For this review, take the finished solid that the model builds, in its own axes (mm). A direction names the side the tool comes from. Give positions to 0.01 mm unless a question says otherwise; leave off trailing zeros. Write each loop counter-clockwise with the first axis right and the second up, starting at its lowest first coordinate (ties: lowest second). Pieces come first, ordered by that corner, then holes. Notation, with made-up numbers: M 20,-29.5 L 77,-29.5 A16 ccw 77,-25.5 Z; hole C 55.25,78.5 d6. An arc over 180 degrees is marked long. Write item = value, one per line.
```python
from build123d import *

# Parameters (mm, degrees)
SKETCH2_W           = 54.6
SKETCH2_H           = 28
SKETCH2_R           = 2.04
SKETCH2_W_2         = 40.6
SKETCH2_H_2         = 20.5
BOSS_EXTRUDE1_DEPTH = 7.5
BOSS_EXTRUDE2_DEPTH = 7.5
BOSS_EXTRUDE3_DEPTH = 40.72
SKETCH6_W           = 18.087587328
SKETCH6_H           = 12.11
SKETCH6_W_2         = 10.871882737
CUT_EXTRUDE2_DEPTH  = 75
CUT_EXTRUDE3_DEPTH  = 24.22
FILLET2_START       = -28.72
FILLET2_DEPTH       = 24.22
FILLET2_START_2     = -3.36744
FILLET2_2_DEPTH     = 11.36744
FILLET2_START_3     = -40.72
FILLET2_3_DEPTH     = 12
FILLET2_START_4     = -4.5
FILLET2_4_DEPTH     = 12
FILLET3_R           = 2
SKETCH8_W           = 25
SKETCH8_H           = 9
SKETCH8_R           = 2.05
BOSS_EXTRUDE4_DEPTH = 7.5
BOSS_EXTRUDE5_DEPTH = 18.75
FILLET5_START       = -59.47
FILLET5_DEPTH       = 18.75
FILLET5_START_2     = -40.72
FILLET5_2_DEPTH     = 12
FILLET5_START_3     = -28.72
FILLET5_3_DEPTH     = 36.72
SKETCH10_R          = 2.05
CUT_EXTRUDE4_DEPTH  = 48.75
SKETCH11_R          = 2.05
CUT_EXTRUDE5_DEPTH  = 13.75


with BuildPart() as part:
    # Sketch2 → Boss-Extrude1 (new body)
    with BuildSketch(Plane.XY):
        Rectangle(SKETCH2_W, SKETCH2_H)
        with Locations((23.85, 4.9)):
            Circle(SKETCH2_R, mode=Mode.SUBTRACT)
        with Locations((23.85, -4.9)):
            Circle(SKETCH2_R, mode=Mode.SUBTRACT)
        with Locations((-23.85, -4.9)):
            Circle(SKETCH2_R, mode=Mode.SUBTRACT)
        with Locations((-23.85, 4.9)):
            Circle(SKETCH2_R, mode=Mode.SUBTRACT)
        Rectangle(SKETCH2_W_2, SKETCH2_H_2, mode=Mode.SUBTRACT)
    extrude(amount=BOSS_EXTRUDE1_DEPTH)

    # Sketch3 → Boss-Extrude2 (add)
    with BuildSketch(Plane.XY.offset(7.5)):
        with BuildLine():
            ThreePointArc((60.895347856, 47.266361721), (62.080408935, 46.696685397), (63.247918809, 46.091853548))
            Line((63.247918809, 46.091853548), (65.410652729, 47.340508558))
            ThreePointArc((65.410652729, 47.340508558), (63.367825291, 52.693526286), (60.533352794, 57.672854393))
            ThreePointArc((60.533352794, 57.672854393), (14.45073797, 52.932517239), (-10.655780842, 14))
            Line((-10.655780842, 14), (27.3, 14))
            Line((27.3, 14), (29.456139987, 36.685790659))
            ThreePointArc((29.456139987, 36.685790659), (31.415329504, 44.731485751), (36.854221074, 50.975690388))
            ThreePointArc((36.854221074, 50.975690388), (38.81261709, 52.175562601), (40.911281353, 53.108630977))
            Line((40.911281353, 53.108630977), (43.979720969, 47.793937662))
            Line((43.979720969, 47.793937662), (43.979720969, 53.930816894))
            ThreePointArc((43.979720969, 53.930816894), (53.370921787, 52.967700083), (60.895347856, 47.266361721))
        make_face()
        with BuildLine():
            ThreePointArc((0.216101895, 19.75), (7.968248239, 34.690697157), (20.76316619, 45.627345599))
            Line((20.76316619, 45.627345599), (18.303689223, 19.75))
            Line((18.303689223, 19.75), (0.216101895, 19.75))
        make_face(mode=Mode.SUBTRACT)
    extrude(amount=-BOSS_EXTRUDE2_DEPTH)

    # Sketch4 → Boss-Extrude3 (add)
    with BuildSketch(Plane(origin=(0, 0, 0), x_dir=(-1, 0, 0), z_dir=(0, 0, -1))):
        with BuildLine():
            Line((-27.3, 14), (10.655780842, 14))
            ThreePointArc((10.655780842, 14), (-14.45073797, 52.932517239), (-60.533352794, 57.672854393))
            ThreePointArc((-60.533352794, 57.672854393), (-63.367825291, 52.693526286), (-65.410652729, 47.340508558))
            Line((-65.410652729, 47.340508558), (-63.247918809, 46.091853548))
            ThreePointArc((-63.247918809, 46.091853548), (-62.080408935, 46.696685397), (-60.895347856, 47.266361721))
            ThreePointArc((-60.895347856, 47.266361721), (-53.370921787, 52.967700083), (-43.979720969, 53.930816894))
            Line((-43.979720969, 53.930816894), (-43.979720969, 47.793937662))
            Line((-43.979720969, 47.793937662), (-40.911281353, 53.108630977))
            ThreePointArc((-40.911281353, 53.108630977), (-32.60282981, 46.697408258), (-29.456139987, 36.685790659))
            Line((-29.456139987, 36.685790659), (-27.3, 14))
        make_face()
        with BuildLine():
            ThreePointArc((-20.76316619, 45.627345599), (-7.968248239, 34.690697157), (-0.216101895, 19.75))
            Line((-0.216101895, 19.75), (-18.303689223, 19.75))
            Line((-18.303689223, 19.75), (-20.76316619, 45.627345599))
        make_face(mode=Mode.SUBTRACT)
    extrude(amount=BOSS_EXTRUDE3_DEPTH)

    # Sketch6 → Cut-Extrude2 (cut)
    with BuildSketch(Plane.XZ.offset(-14)):
        with Locations((9.259895559, -22.665)):
            Rectangle(SKETCH6_W, SKETCH6_H)
        with Locations((9.259895559, -10.555)):
            Rectangle(SKETCH6_W, SKETCH6_H)
        with Locations((-5.219839474, -10.555)):
            Rectangle(SKETCH6_W_2, SKETCH6_H)
        with Locations((-5.219839474, -22.665)):
            Rectangle(SKETCH6_W_2, SKETCH6_H)
    extrude(amount=-CUT_EXTRUDE2_DEPTH, mode=Mode.SUBTRACT)

    # Sketch7 → Cut-Extrude3 (cut)
    with BuildSketch(Plane(origin=(0, 0, -4.5), x_dir=(-1, 0, 0), z_dir=(0, 0, -1))):
        Polygon((-18.303689223, 19.75), (-27.846500896, 19.75), (-54.079071881, 47.777058416), (-54.079071881, 65.656726539), (-18.303689223, 62.002487799), align=None)
    extrude(amount=CUT_EXTRUDE3_DEPTH, mode=Mode.SUBTRACT)

    # Fillet2: read off the stored shape, not the designer's step
    # Fillet2 outline → Fillet2 (cut)
    with BuildSketch(Plane.XY.offset(FILLET2_START)):
        with BuildLine():
            ThreePointArc((55.143386559, 52.15249663), (54.365687709, 52.888463891), (54.079071881, 53.920120169))
            Line((54.079071881, 53.920120169), (54.079071881, 52.670590979))
            ThreePointArc((54.079071881, 52.670590979), (54.615611027, 52.420545294), (55.143386559, 52.15249663))
        make_face()
        with BuildLine():
            ThreePointArc((56.609256937, 58.915929333), (55.348001268, 59.246208749), (54.079071881, 59.545655852))
            Line((54.079071881, 59.545655852), (54.079071881, 56.987483377))
            ThreePointArc((54.079071881, 56.987483377), (54.866712634, 58.57813892), (56.609256937, 58.915929333))
        make_face()
        with BuildLine():
            Line((18.303689223, 19.75), (18.303689223, 17.75))
            ThreePointArc((18.303689223, 17.75), (18.88947566, 19.164213562), (20.303689223, 19.75))
            Line((20.303689223, 19.75), (18.303689223, 19.75))
        make_face()
    extrude(amount=FILLET2_DEPTH, mode=Mode.SUBTRACT)

    # Fillet2 2 outline → Fillet2 2 (cut)
    with BuildSketch(Plane.XY.offset(FILLET2_START_2)):
        with BuildLine():
            Line((-27.3, 14), (-27.3, 12))
            ThreePointArc((-27.3, 12), (-26.714213562, 13.414213562), (-25.3, 14))
            Line((-25.3, 14), (-27.3, 14))
        make_face()
        with BuildLine():
            ThreePointArc((27.3, -12), (26.714213562, -13.414213562), (25.3, -14))
            Line((25.3, -14), (27.3, -14))
            Line((27.3, -14), (27.3, -12))
        make_face()
    extrude(amount=FILLET2_2_DEPTH, mode=Mode.SUBTRACT)

    # Fillet2 3 outline → Fillet2 3 (add)
    with BuildSketch(Plane.XY.offset(FILLET2_START_3)):
        with BuildLine():
            ThreePointArc((17.242809806, 43.409998621), (19.395297177, 43.497545876), (20.378564388, 41.5807642))
            Line((20.378564388, 41.5807642), (20.76316619, 45.627345599))
            ThreePointArc((20.76316619, 45.627345599), (18.976765346, 44.560304331), (17.242809806, 43.409998621))
        make_face()
    extrude(amount=FILLET2_3_DEPTH)

    # Fillet2 4 outline → Fillet2 4 (add)
    with BuildSketch(Plane.XY.offset(FILLET2_START_4)):
        with BuildLine():
            ThreePointArc((17.242809806, 43.409998621), (19.395297177, 43.497545876), (20.378564388, 41.5807642))
            Line((20.378564388, 41.5807642), (20.76316619, 45.627345599))
            ThreePointArc((20.76316619, 45.627345599), (18.976765346, 44.560304331), (17.242809806, 43.409998621))
        make_face()
    extrude(amount=FILLET2_4_DEPTH)

    # Fillet3
    fillet3_edges = [part.edges().sort_by_distance(p)[0] for p in [
        (-10.655780842, 14, 3.75),
    ]]
    fillet(fillet3_edges, radius=FILLET3_R)

    # Sketch8 → Boss-Extrude4 (add)
    with BuildSketch(Plane(origin=(0, 0, 0), x_dir=(-1, 0, 0), z_dir=(0, 0, -1))):
        with Locations((14.8, -18.5)):
            Rectangle(SKETCH8_W, SKETCH8_H)
        with Locations((19.8, -18.5)):
            Circle(SKETCH8_R, mode=Mode.SUBTRACT)
        with Locations(Location((9.8, -18.5, 0), (0, 0, 180))):
            Circle(SKETCH8_R, mode=Mode.SUBTRACT)
    extrude(amount=-BOSS_EXTRUDE4_DEPTH)

    # Sketch9 → Boss-Extrude5 (add)
    with BuildSketch(Plane(origin=(0, 0, -40.72), x_dir=(-1, 0, 0), z_dir=(0, 0, -1))):
        with BuildLine():
            Line((9.611579134, 19.75), (-0.216101895, 19.75))
            Line((-0.216101895, 19.75), (-0.216101895, 14))
            Line((-0.216101895, 14), (10.655780842, 14))
            ThreePointArc((10.655780842, 14), (10.212250908, 16.889268502), (9.611579134, 19.75))
        make_face()
        with BuildLine():
            Line((-27.3, 46.646953525), (-6.144205282, 46.646953525))
            ThreePointArc((-6.144205282, 46.646953525), (-16.03112882, 53.865128552), (-27.3, 58.646953525))
            Line((-27.3, 58.646953525), (-27.3, 46.646953525))
        make_face()
        with BuildLine():
            Line((-54.351959568, 52.546176932), (-57.239489727, 58.738505342))
            ThreePointArc((-57.239489727, 58.738505342), (-58.895043232, 58.232329863), (-60.533352794, 57.672854393))
            ThreePointArc((-60.533352794, 57.672854393), (-63.367825291, 52.693526286), (-65.410652729, 47.340508558))
            Line((-65.410652729, 47.340508558), (-63.247918809, 46.091853548))
            ThreePointArc((-63.247918809, 46.091853548), (-62.080408935, 46.696685397), (-60.895347856, 47.266361721))
            ThreePointArc((-60.895347856, 47.266361721), (-57.945451214, 50.305079876), (-54.351959568, 52.546176932))
        make_face()
    extrude(amount=BOSS_EXTRUDE5_DEPTH)

    # Fillet5: read off the stored shape, not the designer's step
    # Fillet5 outline → Fillet5 (cut)
    with BuildSketch(Plane.XY.offset(FILLET5_START)):
        with BuildLine():
            ThreePointArc((-8.338152673, 14), (-9.866779191, 14.710309738), (-10.309607406, 16.336699029))
            ThreePointArc((-10.309607406, 16.336699029), (-10.49559232, 15.170260335), (-10.655780842, 14))
            Line((-10.655780842, 14), (-8.338152673, 14))
        make_face()
        with BuildLine():
            ThreePointArc((10.489442502, 50.25149541), (8.269243735, 48.506581845), (6.144205282, 46.646953525))
            Line((6.144205282, 46.646953525), (11.683362659, 46.646953525))
            ThreePointArc((11.683362659, 46.646953525), (9.784799548, 48.018098919), (10.489442502, 50.25149541))
        make_face()
        with BuildLine():
            ThreePointArc((-9.96667316, 18.154660194), (-9.271106016, 19.30069668), (-8.008038399, 19.75))
            Line((-8.008038399, 19.75), (-9.611579134, 19.75))
            ThreePointArc((-9.611579134, 19.75), (-9.795218542, 18.953686155), (-9.96667316, 18.154660194))
        make_face()
        with BuildLine():
            ThreePointArc((27.3, 58.646953525), (25.961797954, 58.233374024), (24.634881293, 57.784904523))
            ThreePointArc((24.634881293, 57.784904523), (26.45537063, 57.531258997), (27.3, 55.898739868))
            Line((27.3, 55.898739868), (27.3, 58.646953525))
        make_face()
        with BuildLine():
            ThreePointArc((27.3, 48.646953525), (26.714213562, 47.232739963), (25.3, 46.646953525))
            Line((25.3, 46.646953525), (27.3, 46.646953525))
            Line((27.3, 46.646953525), (27.3, 48.646953525))
        make_face()
    extrude(amount=FILLET5_DEPTH, mode=Mode.SUBTRACT)

    # Fillet5 2 outline → Fillet5 2 (cut)
    with BuildSketch(Plane.XY.offset(FILLET5_START_2)):
        with BuildLine():
            ThreePointArc((-8.338152673, 14), (-9.866779191, 14.710309738), (-10.309607406, 16.336699029))
            ThreePointArc((-10.309607406, 16.336699029), (-10.49559232, 15.170260335), (-10.655780842, 14))
            Line((-10.655780842, 14), (-8.338152673, 14))
        make_face()
    extrude(amount=FILLET5_2_DEPTH, mode=Mode.SUBTRACT)

    # Fillet5 3 outline → Fillet5 3 (cut)
    with BuildSketch(Plane.XY.offset(FILLET5_START_3)):
        with BuildLine():
            Line((-2.3, -23), (-2.3, -21))
            ThreePointArc((-2.3, -21), (-2.885786438, -22.414213562), (-4.3, -23))
            Line((-4.3, -23), (-2.3, -23))
        make_face()
        with BuildLine():
            Line((-27.3, -23), (-25.3, -23))
            ThreePointArc((-25.3, -23), (-26.714213562, -22.414213562), (-27.3, -21))
            Line((-27.3, -21), (-27.3, -23))
        make_face()
    extrude(amount=FILLET5_3_DEPTH, mode=Mode.SUBTRACT)

    # Sketch10 → Cut-Extrude4 (cut)
    with BuildSketch(Plane.XZ.offset(-14)):
        with Locations((-5.061025389, -50.47)):
            Circle(SKETCH10_R)
        with Locations((18.491681329, -50.47)):
            Circle(SKETCH10_R)
    extrude(amount=-CUT_EXTRUDE4_DEPTH, mode=Mode.SUBTRACT)

    # Sketch11 → Cut-Extrude5 (cut)
    with BuildSketch(Plane(origin=(47.112556242, 58.387601913, 0), x_dir=(-0.7782450980918282, 0.6279606415182729, 0), z_dir=(-0.6279606415182729, -0.7782450980918282, 0))):
        with Locations(Location((-14.561184245, 50.47, 0), (0, 0, 180))):
            Circle(SKETCH11_R)
    extrude(amount=-CUT_EXTRUDE5_DEPTH, mode=Mode.SUBTRACT)


solid = part.part
```
1. We need section A-A, the plane y = 1. Write out the cut boundary in (x, z).
Responses:
outline = M -27.3,0 L -20.3,0 L -20.3,7.5 L -27.3,7.5 Z; M 20.3,0 L 27.3,0 L 27.3,7.5 L 20.3,7.5 Z
2. For line 1 along Y through (x, z) = (-23, 1); line 2 along X through (y, z) = (-18, 5); line 3 along Y through (x, z) = (23.85, 4.75), list the stretches that pass through material, from the lowest coordinate up. Write a range as from..to.
Responses:
line_1 = -23..-6.75, -3.05..3.05, 6.75..14
line_2 = -27.3..-21.79, -17.81..-11.79, -7.81..-2.3
line_3 = -14..-6.94, -2.86..2.86, 6.94..57.5
3. Machinability: for faces 1 (the face through (0.216, 17, -50)), 2 (the face through (24, 19.75, -16)), 3 (the face through (0, 10.25, 4)), 4 (the face through (9.796, 47.985, -50.226)), 5 (the face through (26.43, 57.55, -50.23)), which of the approach directions +Z, -Z, +X, -X, +Y, -Y give a long, thin tool a straight path to every point of the face, cutting with its end or side? Answer none if there is none.
Responses:
face_1 = -Z, +X, +Y, -Y
face_2 = +X, -X, +Y
face_3 = +Z, -Z
face_4 = -Z, -X
face_5 = -Z, +Y
4. The part is to be moulded in two halves that separate along Z. For faces 6 (the face through (32.69, 46.82, -34.64)), 7 (the face through (21, 51, -59.47)), 8 (the face through (20.385, 51.331, -51.255)), say which applies: +Z half, -Z half, draft (parallel to the pull), parting line (faces both ways), or undercut.
Responses:
face_6 = draft
face_7 = -Z half
face_8 = undercut
5. We need section B-B, the plane z = -35.5. Write out the cut boundary in (x, y).
Responses:
outline = M -10.31,16.34 A2 ccw -8.34,14 L 27.3,14 L 29.46,36.69 A17.5 cw 40.91,53.11 L 43.98,47.79 L 43.98,53.93 A17.5 cw 60.9,47.27 A44 cw 63.25,46.09 L 65.41,47.34 A37.5 ccw 60.53,57.67 A53.5 ccw Z; hole M 0.22,19.75 L 18.3,19.75 L 20.38,41.58 A2 ccw 17.24,43.41 A44 ccw Z
6. We need section D-D, the plane z = -43. Write out the cut boundary in (x, y).
Responses:
outline = M -10.31,16.34 A2 ccw -8.34,14 L 0.22,14 L 0.22,19.75 L -8.01,19.75 A2 ccw -9.97,18.15 A53.5 ccw Z; M 10.49,50.25 A2 ccw 11.68,46.65 L 25.3,46.65 A2 ccw 27.3,48.65 L 27.3,55.9 A2 ccw 24.63,57.78 A53.5 ccw Z; M 54.35,52.55 A17.5 cw 60.9,47.27 A44 cw 63.25,46.09 L 65.41,47.34 A37.5 ccw 60.53,57.67 A53.5 ccw 57.24,58.74 Z
7. We need section C-C, the plane x = -23.85. Write out the cut boundary in (y, z), then the cut area to 3 significant figures.
Responses:
outline = M -23,0 L -6.94,0 L -6.94,7.5 L -23,7.5 Z; M -2.86,0 L 2.86,0 L 2.86,7.5 L -2.86,7.5 Z; M 6.94,0 L 14,0 L 14,7.5 L 6.94,7.5 Z
area = 216 mm2
8. Insertion check: P1, Ø12, axis at x = -2.5, z = -42.5, coming from the -Y side; P2, Ø8, axis at x = -20, z = 4, coming from the +Y side; P3, Ø12, axis at y = 37.5, z = -31, coming from the -X side. Each pin has a flat end and moves straight along its axis. Give the tip position at first contact, or say it passes through.
Responses:
P1 = 14
P2 = 14
P3 = -5.3
